Geometry: final body of the model. Coordinates: model frame, mm. A direction names the side the tool comes from. Give positions to 0.01 mm unless a question says otherwise; leave off trailing zeros. Loops run counter-clockwise (first coordinate to the right, second up) from the corner with the lowest first, then second, coordinate; pieces in that order, holes last.
from build123d import *

# Parameters (mm, degrees)
SKETCH1_W           = 51
SKETCH1_H           = 62
BOSS_EXTRUDE1_DEPTH = 7
SKETCH2_W           = 29
SKETCH2_H           = 21
CUT_EXTRUDE1_DEPTH  = 8
SKETCH9_R           = 1.75
CUT_EXTRUDE4_DEPTH  = 8
CUT_EXTRUDE5_DEPTH  = 8
BOSS_EXTRUDE4_DEPTH = 10
SKETCH13_R          = 1.75
CUT_EXTRUDE6_DEPTH  = 63
FILLET1_R           = 3


with BuildPart() as part:
    # Sketch1 → Boss-Extrude1 (new body)
    with BuildSketch(Plane(origin=(0, 0, 0), x_dir=(1, 0, 0), z_dir=(0, 1, 0))):
        with Locations((25.5, 31)):
            Rectangle(SKETCH1_W, SKETCH1_H)
    extrude(amount=BOSS_EXTRUDE1_DEPTH)

    # Sketch2 → Cut-Extrude1 (cut, through all)
    with BuildSketch(Plane(origin=(0, 7, 0), x_dir=(1, 0, 0), z_dir=(0, 1, 0))):
        with Locations((25.5, 51.5)):
            Rectangle(SKETCH2_W, SKETCH2_H)
    extrude(amount=-CUT_EXTRUDE1_DEPTH, mode=Mode.SUBTRACT)

    # Sketch9 → Cut-Extrude4 (cut, through all)
    with BuildSketch(Plane(origin=(0, 7, 0), x_dir=(1, 0, 0), z_dir=(0, 1, 0))):
        with Locations((5.5, 54)):
            Circle(SKETCH9_R)
        with Locations((45.5, 54)):
            Circle(SKETCH9_R)
    extrude(amount=-CUT_EXTRUDE4_DEPTH, mode=Mode.SUBTRACT)

    # Sketch11 → Cut-Extrude5 (cut, through all)
    with BuildSketch(Plane(origin=(0, 7, 0), x_dir=(1, 0, 0), z_dir=(0, 1, 0))):
        Polygon((20.5, 0), (0, 31), (0, 0), align=None)
        Polygon((30.5, 0), (51, 31), (51, 0), align=None)
    extrude(amount=-CUT_EXTRUDE5_DEPTH, mode=Mode.SUBTRACT)

    # Sketch12 → Boss-Extrude4 (add)
    with BuildSketch(Plane(origin=(0, 7, 0), x_dir=(1, 0, 0), z_dir=(0, 1, 0))):
        Polygon((30.5, 0), (20.5, 0), (15.870967742, 7), (35.129032258, 7), align=None)
    boss_extrude4 = extrude(amount=BOSS_EXTRUDE4_DEPTH)

    # Mirror1: Boss-Extrude4 across plane
    add(boss_extrude4.mirror(Plane.ZX.offset(3.5)))

    # Sketch13 → Cut-Extrude6 (cut, through all)
    with BuildSketch(Plane.XY):
        with Locations((25.5, 13.5)):
            Circle(SKETCH13_R)
        with Locations((25.5, -6.5)):
            Circle(SKETCH13_R)
    extrude(amount=-CUT_EXTRUDE6_DEPTH, mode=Mode.SUBTRACT)

    # Fillet1
    fillet1_edges = [part.edges().sort_by_distance(p)[0] for p in [
        (25.5, 7, -7),
        (25.5, 0, -7),
    ]]
    fillet(fillet1_edges, radius=FILLET1_R)


solid = part.part
Item 1: Ray query, probe 1 along X at (y, z) = (4.75, -54); probe 2 along X at (y, z) = (0.75, -52.5); probe 3 along Z at (x, y) = (23, -7.75). Return the intervals inside material, ascending.
Values follow:
probe 1: x = 0 to 3.75, 7.25 to 11, 40 to 43.75, 47.25 to 51
probe 2: x = 0 to 4.6, 6.4 to 11, 40 to 44.6, 46.4 to 51
probe 3: z = -7 to 0
Item 2: Pin query (flat end, axial travel): pin 1 (3 mm diameter, centred on x = 15, y = 12.5, fed in from -Z); pin 2 (10 mm diameter, centred on x = 40.5, z = -40.5, fed in from -Y); pin 3 (7.5 mm diameter, centred on x = 30, y = 3.5, fed in from -Z). Return the tip coordinate at first contact, or that it passes through.
Values follow:
pin 1: stops at z = -7
pin 2: stops at y = 0
pin 3: stops at z = -41
Item 3: Section query C-C on x = 23. Return loops of the section in (y, z).
Values follow:
outline: (-10, -7) - (-3, -7) arc R3 cw to (0, -10) - (0, -41) - (7, -41) - (7, -10) arc R3 cw to (10, -7) - (17, -7) - (17, 0) - (-10, 0) - close
Item 4: Section query B-B on z = -57. Return loops of the section in (x, y), plus the area to 3 significant figures.
Values follow:
outline: (0, 0) - (11, 0) - (11, 7) - (0, 7) - close; (40, 0) - (51, 0) - (51, 7) - (40, 7) - close
area: 154 mm2
Item 5: Section query A-A on y = -6.5. Return loops of the section in (x, z), plus the area to 3 significant figures.
Values follow:
outline: (15.87, -7) - (23.75, -7) - (23.75, 0) - (20.5, 0) - close; (27.25, -7) - (35.13, -7) - (30.5, 0) - (27.25, 0) - close
area: 77.9 mm2
Item 6: Section query D-D on z = -37. Return loops of the section in (x, y).
Values follow:
outline: (0, 0) - (51, 0) - (51, 7) - (0, 7) - close
Item 7: Draft query along X for faces 1 (the face through (51, 3, -46)), 2 (the face through (25, 4, -41)), 3 (the face through (40, 4, -51)), 4 (the face through (28, -6, -7)). Return one class per face: +X half, -X half, draft (parallel to the pull), parting line (faces both ways), or undercut.
Values follow:
face 1: +X half
face 2: undercut
face 3: undercut
face 4: draft
Item 8: Set-up query: faces 5 (the face through (47.117, 3.549, -53.33)), 6 (the face through (25, 0, -36)), 7 (the face through (11, 4, -51)), 8 (the face through (25, 7, -36)), 9 (the face through (45, 3, -62)). Return all of +Z, -Z, +X, -X, +Y, -Y with unobstructed straight access to the full face (end or side cutting, diameter ignored); none if empty.
Values follow:
face 5: +Y, -Y
face 6: -Z, +X, -X, -Y
face 7: -Z, +Y, -Y
face 8: -Z, +X, -X, +Y
face 9: -Z, +X, -X, +Y, -Y
